Check sheet for the modelled part. Datum: model origin and axes. Units: mm. A direction names the side the tool comes from. Round coordinates to 2 decimals unless told otherwise and drop trailing zeros. Write each loop counter-clockwise with the first axis right and the second up, starting at its lowest first coordinate (ties: lowest second). Pieces come first, ordered by that corner, then holes. Notation, with made-up numbers: (55, -23) - (86, -23) arc R17 cw to (86, -13) - close; hole circle Ø5 at (69, 73). An arc over 180 degrees is marked (long way). Answer as a JSON object with one key per item and string values. Group by question number.
Item 1: Thickness scan on line 1 (Y direction, x = -0.5, z = 2.85); line 2 (Y direction, x = -2, z = 1.35); line 3 (Z direction, x = -7.25, y = -0.25). Record the ranges inside material, lowest first.
Item 2: Sectioned sample at A-A on x = -0.5. Record the boundary of the cut face in (y, z), plus the area to 3 significant figures.
Item 3: Sectioned sample at B-B on z = 0.8. Count the separate pieces of the cut face and the enclosed holes in it, plus the area to 3 significant figures.
Item 4: Release check for a two-part mould opening along Y. For faces 4 (the flat face through (2, -7, 1.7)), 5 (the flat face through (2, -7.5, 1.5)), 6 (the flat face through (-13, -2.3, 1)), 7 (the cylindrical face through (9.07, 3.11, 2.49)) record: pulls with the +Y half, pulls with the -Y half, needs draft (parallel to the pull), parting line crosses it, or undercut.
Item 5: Sectioned sample at D-D on x = -6.5. Record the boundary of the cut face in (y, z), plus the area to 3 significant figures.
Item 6: Set-up check for faces 1 (the cylindrical face through (-12.699, -2.015, 0.986)), 2 (the flat face through (13.5, -4.3, 0.8)), 3 (the flat face through (0.4, 4.6, 2.5)): record each of +Z, -Z, +X, -X, +Y, -Y from which the full face is reachable in a straight line by a thin tool's end or side.
Item 7: Gauge pin test, flat ends, axial feed: P1, Ø0.5, axis at x = 13.5, z = 0.5, coming from the -Y side; P2, Ø0.5, axis at y = -7.5, z = 1, coming from the -X side; P3, Ø2.5, axis at x = -0.5, y = 5.5, coming from the +Z side. Record the tip position at first contact, or that the pin passes through.
Item 8: Sectioned sample at C-C on y = 0.25. Record the boundary of the cut face in (x, z), plus the area to 3 significant figures.
```python
from build123d import *

# Parameters (mm, degrees)
DODANIE_WYCI_GNI_CIE1_DEPTH = 3
WYTNIJ_WYCI_GNI_CIE1_DEPTH  = 2
WYTNIJ_WYCI_GNI_CIE2_REACH  = 30
SZKIC3_W                    = 1.5
SZKIC3_H                    = 1
WYTNIJ_WYCI_GNI_CIE3_REACH  = 18
SZKIC4_W                    = 1
SZKIC4_H                    = 1.5
SZKIC5_R                    = 2
WYTNIJ_WYCI_GNI_CIE4_DEPTH  = 0.5
WYTNIJ_WYCI_GNI_CIE5_REACH  = 4.5
SZKIC6_R                    = 1


with BuildPart() as part:
    # Szkic1 → Dodanie-wyciągnięcie1 (new body)
    with BuildSketch(Plane.XY):
        with BuildLine():
            Line((-11, 8), (8.3, 8))
            Line((8.3, 8), (8.3, 5))
            ThreePointArc((8.3, 5), (9.090811691, 3.090811691), (11, 2.3))
            Line((11, 2.3), (14, 2.3))
            Line((14, 2.3), (14, -5))
            ThreePointArc((14, -5), (13.121320344, -7.121320344), (11, -8))
            Line((11, -8), (-8.3, -8))
            Line((-8.3, -8), (-8.3, -5))
            ThreePointArc((-8.3, -5), (-9.090811691, -3.090811691), (-11, -2.3))
            Line((-11, -2.3), (-14, -2.3))
            Line((-14, -2.3), (-14, 5))
            ThreePointArc((-14, 5), (-13.121320344, 7.121320344), (-11, 8))
        make_face()
    extrude(amount=DODANIE_WYCI_GNI_CIE1_DEPTH)

    # Szkic2 → Wytnij-wyciągnięcie1 (cut)
    with BuildSketch(Plane(origin=(0, 0, 0), x_dir=(-1, 0, 0), z_dir=(0, 0, -1))):
        with BuildLine():
            Line((11, 7), (-7.3, 7))
            ThreePointArc((-7.3, 7), (-8.007106781, 6.707106781), (-8.3, 6))
            Line((-8.3, 6), (-8.3, 5))
            ThreePointArc((-8.3, 5), (-9.090811691, 3.090811691), (-11, 2.3))
            Line((-11, 2.3), (-12, 2.3))
            ThreePointArc((-12, 2.3), (-12.707106781, 2.007106781), (-13, 1.3))
            Line((-13, 1.3), (-13, -5))
            ThreePointArc((-13, -5), (-12.414213562, -6.414213562), (-11, -7))
            Line((-11, -7), (7.3, -7))
            ThreePointArc((7.3, -7), (8.007106781, -6.707106781), (8.3, -6))
            Line((8.3, -6), (8.3, -5))
            ThreePointArc((8.3, -5), (9.090811691, -3.090811691), (11, -2.3))
            Line((11, -2.3), (12, -2.3))
            ThreePointArc((12, -2.3), (12.707106781, -2.007106781), (13, -1.3))
            Line((13, -1.3), (13, 5))
            ThreePointArc((13, 5), (12.414213562, 6.414213562), (11, 7))
        make_face()
    extrude(amount=-WYTNIJ_WYCI_GNI_CIE1_DEPTH, mode=Mode.SUBTRACT)

    # Szkic3 → Wytnij-wyciągnięcie2 (cut, up to next)
    with BuildSketch(Plane(origin=(14, 0, 0), x_dir=(0, 0, -1), z_dir=(1, 0, 0)), mode=Mode.PRIVATE) as wytnij_wyci_gni_cie2_sk1:
        with Locations((-0.75, 1.6)):
            Rectangle(SZKIC3_W, SZKIC3_H)
    wytnij_wyci_gni_cie2_tool1 = extrude(wytnij_wyci_gni_cie2_sk1.sketch, amount=-WYTNIJ_WYCI_GNI_CIE2_REACH, mode=Mode.PRIVATE) & part.part
    add(wytnij_wyci_gni_cie2_tool1.solids().sort_by_distance((14, 1.6, 0.75))[0], mode=Mode.SUBTRACT)
    # Szkic3 → Wytnij-wyciągnięcie2 (cut, up to next)
    with BuildSketch(Plane(origin=(14, 0, 0), x_dir=(0, 0, -1), z_dir=(1, 0, 0)), mode=Mode.PRIVATE) as wytnij_wyci_gni_cie2_sk2:
        with Locations((-0.75, -3.8)):
            Rectangle(SZKIC3_W, SZKIC3_H)
    wytnij_wyci_gni_cie2_tool2 = extrude(wytnij_wyci_gni_cie2_sk2.sketch, amount=-WYTNIJ_WYCI_GNI_CIE2_REACH, mode=Mode.PRIVATE) & part.part
    add(wytnij_wyci_gni_cie2_tool2.solids().sort_by_distance((14, -3.8, 0.75))[0], mode=Mode.SUBTRACT)

    # Szkic4 → Wytnij-wyciągnięcie3 (cut, up to next)
    with BuildSketch(Plane.XZ.offset(8), mode=Mode.PRIVATE) as wytnij_wyci_gni_cie3_sk1:
        with Locations((2, 0.75)):
            Rectangle(SZKIC4_W, SZKIC4_H)
    wytnij_wyci_gni_cie3_tool1 = extrude(wytnij_wyci_gni_cie3_sk1.sketch, amount=-WYTNIJ_WYCI_GNI_CIE3_REACH, mode=Mode.PRIVATE) & part.part
    add(wytnij_wyci_gni_cie3_tool1.solids().sort_by_distance((2, -8, 0.75))[0], mode=Mode.SUBTRACT)

    # Szkic5 → Wytnij-wyciągnięcie4 (cut)
    with BuildSketch(Plane.XY.offset(3)):
        with Locations((-0.5, 5.5)):
            Circle(SZKIC5_R)
    extrude(amount=-WYTNIJ_WYCI_GNI_CIE4_DEPTH, mode=Mode.SUBTRACT)

    # Szkic6 → Wytnij-wyciągnięcie5 (cut, up to next)
    with BuildSketch(Plane.XY.offset(2.5), mode=Mode.PRIVATE) as wytnij_wyci_gni_cie5_sk1:
        with Locations((-0.5, 5.5)):
            Circle(SZKIC6_R)
    wytnij_wyci_gni_cie5_tool1 = extrude(wytnij_wyci_gni_cie5_sk1.sketch, amount=-WYTNIJ_WYCI_GNI_CIE5_REACH, mode=Mode.PRIVATE) & part.part
    add(wytnij_wyci_gni_cie5_tool1.solids().sort_by_distance((-0.5, 5.5, 2.5))[0], mode=Mode.SUBTRACT)


solid = part.part
```
Completed:
{
 "1": {"line 1": "-8 to 3.5, 7.5 to 8", "line 2": "-8 to -7, 7 to 8", "line 3": "2 to 3"},
 "2": {"outline": "(-8, 0) - (-7, 0) - (-7, 2) - (4.5, 2) - (4.5, 2.5) - (3.5, 2.5) - (3.5, 3) - (-8, 3) - close; (6.5, 2) - (7, 2) - (7, 0) - (8, 0) - (8, 3) - (7.5, 3) - (7.5, 2.5) - (6.5, 2.5) - close", "area": "17.0 mm²"},
 "3": {"separate pieces": "5", "enclosed holes": "0", "area": "58.8 mm²"},
 "4": {"face 4": "undercut", "face 5": "needs draft", "face 6": "pulls with the -Y half", "face 7": "pulls with the +Y half"},
 "5": {"outline": "(-8, 0) - (-7, 0) - (-7, 2) - (7, 2) - (7, 0) - (8, 0) - (8, 3) - (-8, 3) - close", "area": "20.0 mm²"},
 "6": {"face 1": "-Z", "face 2": "-Z, +X, -X", "face 3": "+Z"},
 "7": {"P1": "y = -6.98", "P2": "x = -8.3", "P3": "z = 2.5"},
 "8": {"outline": "(-14, 0) - (-13, 0) - (-13, 2) - (13, 2) - (13, 0) - (14, 0) - (14, 3) - (-14, 3) - close", "area": "32.0 mm²"}
}
